Answer from the drawing. Dimensions are ordinates in mm from the lowest x, y and z of the part. A direction names the side the tool comes from. Round coordinates to 2 decimals unless told otherwise and drop trailing zeros. Write each loop counter-clockwise with the first axis right and the second up, starting at its lowest first coordinate (ties: lowest second). Pieces come first, ordered by that corner, then holes.
1. A flat-ended cylindrical pin translates along its axis: pin 1 Ø2 at (x, z) = (41.5, 7) entering from +Y. Find the tip coordinate at first contact, or state that the pin passes through.
2. Find section A-A (y = 1.15). Write down the section's boundary in (x, z).
3. Find section D-D (x = 8). Write down the section's boundary in (y, z), and give its area (3 significant figures).
4. Find section B-B (x = 40.5). Write down the section's boundary in (y, z).
5. A tool of negligible diameter and unlimited length cuts with its end or side. For the marked faces 1 and 2, from which of +Z, -Z, +X, -X, +Y, -Y can it reach the whole face along a straight path? Write none if from no direction.
6. Find section C-C (z = 9). Write down the section's boundary in (x, y), and give its area (3 significant figures).
7. Straight lines are drawn through the part: probe 1 along Y at (x, z) = (37, 1.25); probe 2 along Z at (x, y) = (50, 0.9). For each, find the intervals that lie inside material, in ascending order.
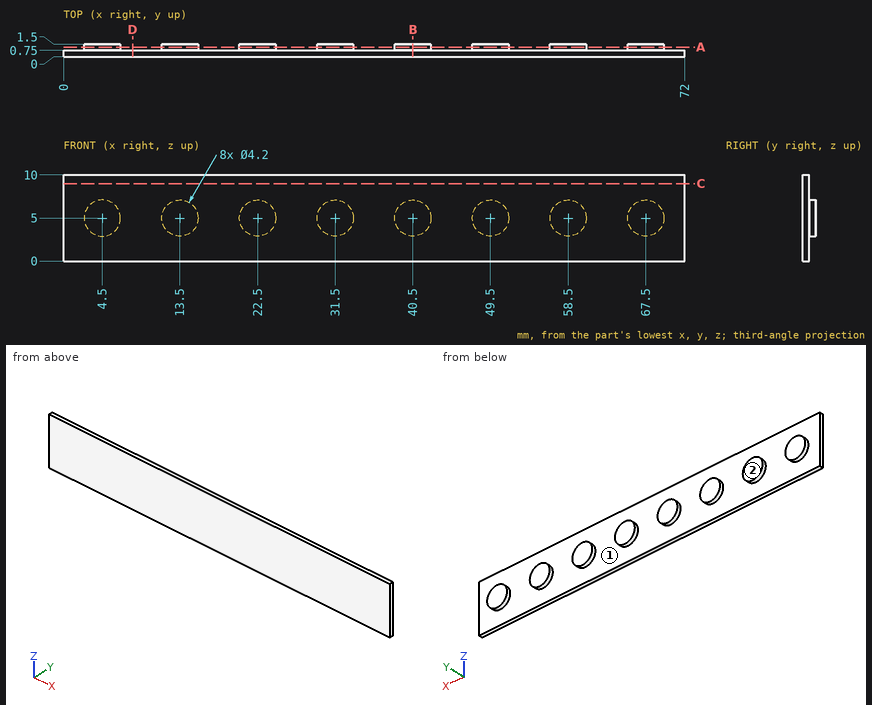
Worked answers:
1. pin 1: stops at y = 1.5
2. outline: circle Ø4.2 at (4.5, 5); circle Ø4.2 at (13.5, 5); circle Ø4.2 at (22.5, 5); circle Ø4.2 at (31.5, 5); circle Ø4.2 at (40.5, 5); circle Ø4.2 at (49.5, 5); circle Ø4.2 at (58.5, 5); circle Ø4.2 at (67.5, 5)
3. outline: (0, 0) - (0.75, 0) - (0.75, 10) - (0, 10) - close
3. area: 7.50 mm2
4. outline: (0, 0) - (0.75, 0) - (0.75, 2.9) - (1.5, 2.9) - (1.5, 7.1) - (0.75, 7.1) - (0.75, 10) - (0, 10) - close
5. face 1: +Y
5. face 2: +Z, -Z, +X, -X, +Y
6. outline: (0, 0) - (72, 0) - (72, 0.75) - (0, 0.75) - close
6. area: 54.0 mm2
7. probe 1: y = 0 to 0.75
7. probe 2: z = 2.96 to 7.04
